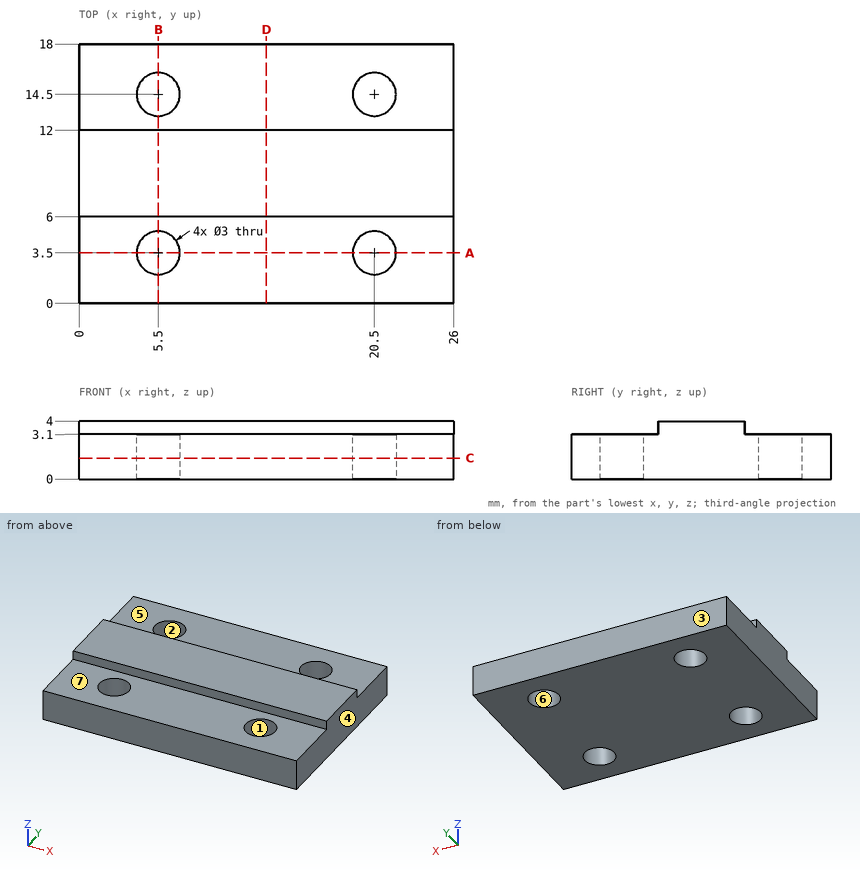
The figure shows three views and two pictorial views of one solid part (mm, origin at its lowest corner). Answer the questions. A direction names the side the tool comes from. Coordinates: 2 decimals unless noted, no trailing zeros. Loops run counter-clockwise (first coordinate to the right, second up) from the corner with the lowest first, then second, coordinate; pieces in that order, holes last. Notation, with made-up numbers: M -38,-35.75 L -31,-35.75 A11 cw -31,-27.75 Z; hole C 38.5,44 d9. An arc over 180 degrees is marked long. Use CSV: the item, a comma, the result in double quotes. Start each with the question number.
(1) Find section C-C, the plane z = 1.45. Give the vertices of the cut face in (x, y), then the cut area to 3 significant figures.
(2) For the marked faces 5, 6 and 7, determine the directions among +Z, -Z, +X, -X, +Y, -Y from which every point of the face is accessible in a straight line to the end or side of a thin tool.
(3) For a pull along Y with two mould halves and no side action, classify the marked faces 1, 2, 3 and 4 as +Y half, -Y half, draft (parallel to the pull), parting line (faces both ways), or undercut.
(4) Find section D-D, the plane x = 13. Give the vertices of the cut face in (y, z), then the cut area to 3 significant figures.
(5) Given pin 1 Ø0.7 at (x, z) = (17.5, 3.5) entering from +Y; pin 2 Ø6.5 at (x, y) = (8, 15.5) entering from +Z, each flat-ended and moving along its own axis, determine where each tip first touches the part or whether it passes through.
(6) Consider line 1 (Y direction, x = 5.5, z = 2.05); line 2 (X direction, y = 2.5, z = 2.45); line 3 (Y direction, x = 19.25, z = 0.55). Determine where each line is inside the solid, lowest interval first.
(7) Find section B-B, the plane x = 5.5. Give the vertices of the cut face in (y, z), then the cut area to 3 significant figures.
(8) Find section A-A, the plane y = 3.5. Give the vertices of the cut face in (x, z).
Recorded:
1,outline,"M 0,0 L 26,0 L 26,18 L 0,18 Z; hole C 5.5,3.5 d3; hole C 5.5,14.5 d3; hole C 20.5,3.5 d3; hole C 20.5,14.5 d3"
1,area,"440 mm^2"
2,face 5,"+Z, +X, -X, +Y"
2,face 6,"+Z, -Z"
2,face 7,"+Z, +X, -X, -Y"
3,face 1,"undercut"
3,face 2,"undercut"
3,face 3,"+Y half"
3,face 4,"draft"
4,outline,"M 0,0 L 18,0 L 18,3.1 L 12,3.1 L 12,4 L 6,4 L 6,3.1 L 0,3.1 Z"
4,area,"61.2 mm^2"
5,pin 1,"stops at y = 12"
5,pin 2,"stops at z = 3.1"
6,line 1,"y = 0 to 2, 5 to 13, 16 to 18"
6,line 2,"x = 0 to 4.38, 6.62 to 19.38, 21.62 to 26"
6,line 3,"y = 0 to 2.67, 4.33 to 13.67, 15.33 to 18"
7,outline,"M 0,0 L 2,0 L 2,3.1 L 0,3.1 Z; M 5,0 L 13,0 L 13,3.1 L 12,3.1 L 12,4 L 6,4 L 6,3.1 L 5,3.1 Z; M 16,0 L 18,0 L 18,3.1 L 16,3.1 Z"
7,area,"42.6 mm^2"
8,outline,"M 0,0 L 4,0 L 4,3.1 L 0,3.1 Z; M 7,0 L 19,0 L 19,3.1 L 7,3.1 Z; M 22,0 L 26,0 L 26,3.1 L 22,3.1 Z"
